Autodesk Inventor part; units mm, degrees
ref_plane "YZ Plane" through (0, 0, 0) normal (1, 0, 0) x (0, 1, 0)
ref_plane "XZ Plane" through (0, 0, 0) normal (0, 1, 0) x (-1, 0, 0)
ref_plane "XY Plane" through (0, 0, 0) normal (0, 0, 1) x (1, 0, 0)
sketch "Boceto1" plane through (0, 0, 0) normal (1, 0, 0) x (0, 1, 0)
  line L0 (1.5, -11.1496) -> (1.5, -13.0893)
  line L1 (-1.5, -11.1496) -> (-1.5, -13.0893)
  line L2 (-1.5, 11.1496) -> (-1.5, 13.0893)
  line L3 (1.5, 11.1496) -> (1.5, 13.0893)
  arc A0 (1.5, 13.0893) -> (-1.5, 13.0893) centre (0, 0) ccw
  arc A1 (-1.5, -13.0893) -> (1.5, -13.0893) centre (0, 0) ccw
  arc A2 (-1.5, 11.1496) -> (-1.5, -11.1496) centre (0, 0) ccw
  arc A3 (1.5, -11.1496) -> (1.5, 11.1496) centre (0, 0) ccw
extrude "Extrusión1" add sketch "Boceto1" along normal blind 3
sketch "Boceto2" plane through (3, 0, 0) normal (1, 0, 0) x (0, 0, -1)
  circle A0 centre (0, 8) radius 1.5
  circle A1 centre (0, -8) radius 1.5
  dimension "d14" = 3
  dimension "d15" = 3
extrude "Extrusión2" cut sketch "Boceto2" against normal blind 3
sketch "Boceto3" plane through (3, 0, 0) normal (1, 0, 0) x (0, 0, -1)
  circle A0 centre (0, 0) radius 1.5
  dimension "d18" = 3
extrude "Extrusión3" cut sketch "Boceto3" against normal blind 10
properties part number "tapa"
Could you check a few things on this model? Use its own coordinates, in mm. A direction names the side the tool comes from. Give positions to 0.01 mm unless a question says otherwise; leave off trailing zeros. Order: outer loops, then holes, each group sorted by start corner. A loop starts at its lowest first (then second) coordinate and runs counter-clockwise, first axis right, second up. Notation, with made-up numbers: (-12.75, -36.75) - (45.25, -36.75) arc R11 ccw to (45.25, -26.75) - close; hole circle Ø10 at (-25, 89.25). An arc over 180 degrees is marked (long way). Return JSON: item names as keys, results as strings. Group by question number.
Q1. Suppose I cut it at B-B, the plane x = 1.2. Please give me the cut outline in (y, z).
Q2. Please list where these lines run through material, in increasing order: line 1 along Y through (x, z) = (1.55, -0.75); line 2 along Y through (x, z) = (2.2, -1.25); line 3 along Z through (x, y) = (2.4, -8.75). Write a range as [from, to].
Q3. Suppose I cut it at D-D, the plane z = 4.5. Please give me the cut outline in (x, y), and give its area (3 significant figures).
Q4. Which directions (+Z, -Z, +X, -X, +Y, -Y) give clear straight access to the entire face, cutting with the end or side of a thin tool? Please do faces 4 (the face through (0, 2, 0)), 5 (the face through (1, -1.5, 12)), 6 (the face through (1, 1.5, 12)).
Q5. Will these pins go through, and if not, where does the flat tip stop? pin 1 Ø1.6 at (x, z) = (2, 12.5) entering from -Y; pin 2 Ø0.6 at (x, z) = (1.5, 12) entering from +Y.
Q6. Suppose I cut it at C-C, the plane y = 7. Please give me the cut outline in (x, z).
Q7. Thinking about a two-plate mould opening in Y: for faces 1 (the face through (1.521, -9.464, 0.325)), 2 (the face through (1, -1.5, -12)), 3 (the face through (1, 1.5, -12)), which applies, pulls with the +Y half, pulls with the -Y half, needs draft (parallel to the pull), parting line crosses it, or undercut?
Q8. Suppose I cut it at A-A, the plane y = 0. Please give me the cut outline in (x, z), and give its area (4 significant figures).
Resolved:
{
 "1": {"outline": "(-1.5, -13.09) arc R13.17 ccw to (1.5, -13.09) - (1.5, -11.15) arc R11.25 ccw to (1.5, 11.15) - (1.5, 13.09) arc R13.17 ccw to (-1.5, 13.09) - (-1.5, 11.15) arc R11.25 ccw to (-1.5, -11.15) - close; hole circle Ø3 at (-8, 0); hole circle Ø3 at (0, 0); hole circle Ø3 at (8, 0)"},
 "2": {"line 1": "y = [-11.23, -9.3], [-6.7, -1.3], [1.3, 6.7], [9.3, 11.23]", "line 2": "y = [-11.18, -8.83], [-7.17, -0.83], [0.83, 7.17], [8.83, 11.18]", "line 3": "z = [-7.07, -1.3], [1.3, 7.07]"},
 "3": {"outline": "(0, -10.31) - (3, -10.31) - (3, 10.31) - (0, 10.31) - close", "area": "61.9 mm2"},
 "4": {"face 4": "+Z, -Z, -X, +Y, -Y", "face 5": "+Z, +X, -X, -Y", "face 6": "+Z, +X, -X, +Y"},
 "5": {"pin 1": "stops at y = -1.5", "pin 2": "stops at y = 1.5"},
 "6": {"outline": "(0, -8.81) - (3, -8.81) - (3, -1.12) - (0, -1.12) - close; (0, 1.12) - (3, 1.12) - (3, 8.81) - (0, 8.81) - close"},
 "7": {"face 1": "undercut", "face 2": "pulls with the -Y half", "face 3": "pulls with the +Y half"},
 "8": {"outline": "(0, -13.17) - (3, -13.17) - (3, -1.5) - (0, -1.5) - close; (0, 1.5) - (3, 1.5) - (3, 13.17) - (0, 13.17) - close", "area": "70.05 mm2"}
}
